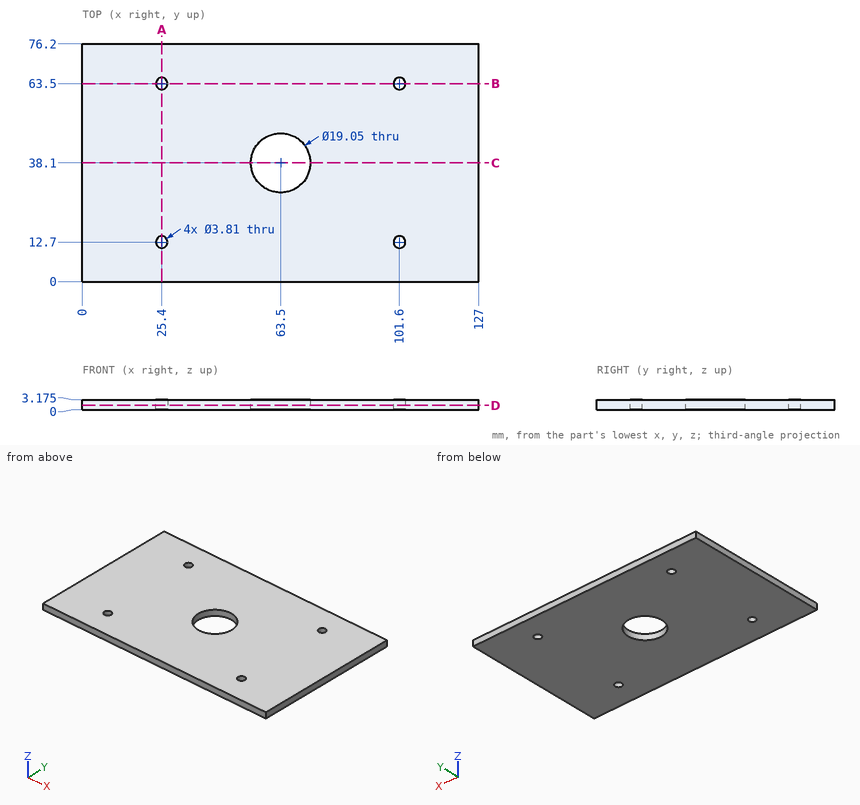
Answer from the drawing. Dimensions are ordinates in mm from the lowest x, y and z of the part. Round coordinates to 2 decimals unless told otherwise and drop trailing zeros. Order: outer loops, then holes, each group sorted by start corner. A loop starts at its lowest first (then second) coordinate and runs counter-clockwise, first axis right, second up.
1) The part is cut by section A-A on x = 25.4. Write down the section's boundary in (y, z) (3 decimals).
2) The part is cut by section C-C on y = 38.1. Write down the section's boundary in (x, z) (3 decimals).
3) Straight lines are drawn through the part: L1, parallel to Y at x = 25.4, z = 2.45 (3 decimals); L2, parallel to Y at x = 63.5, z = 2.1 (3 decimals); L3, parallel to Y at x = 103, z = 0.3. For each, find the intervals that lie inside material, in ascending order.
4) The part is cut by section D-D on z = 1.35. Write down the section's boundary in (x, y) (3 decimals), plus the area to 3 significant figures.
5) The part is cut by section B-B on y = 63.5. Write down the section's boundary in (x, z) (3 decimals).
Resolved:
1. outline: (0, 0) - (10.795, 0) - (10.795, 3.175) - (0, 3.175) - close; (14.605, 0) - (61.595, 0) - (61.595, 3.175) - (14.605, 3.175) - close; (65.405, 0) - (76.2, 0) - (76.2, 3.175) - (65.405, 3.175) - close
2. outline: (0, 0) - (53.975, 0) - (53.975, 3.175) - (0, 3.175) - close; (73.025, 0) - (127, 0) - (127, 3.175) - (73.025, 3.175) - close
3. L1: y = 0 to 10.795, 14.605 to 61.595, 65.405 to 76.2
3. L2: y = 0 to 28.575, 47.625 to 76.2
3. L3: y = 0 to 11.41, 13.99 to 62.21, 64.79 to 76.2
4. outline: (0, 0) - (127, 0) - (127, 76.2) - (0, 76.2) - close; hole circle Ø3.81 at (25.4, 12.7); hole circle Ø3.81 at (25.4, 63.5); hole circle Ø19.05 at (63.5, 38.1); hole circle Ø3.81 at (101.6, 12.7); hole circle Ø3.81 at (101.6, 63.5)
4. area: 9,350 mm2
5. outline: (0, 0) - (23.495, 0) - (23.495, 3.175) - (0, 3.175) - close; (27.305, 0) - (99.695, 0) - (99.695, 3.175) - (27.305, 3.175) - close; (103.505, 0) - (127, 0) - (127, 3.175) - (103.505, 3.175) - close
